Here's the drawing with two shaded views (mm, measured from the low corner). I have some questions. Give positions to 0.01 mm unless a question says otherwise; leave off trailing zeros. Order: outer loops, then holes, each group sorted by start corner. A loop starts at its lowest first (then second) coordinate and runs counter-clockwise, first axis right, second up. Notation, with made-up numbers: M -28,-38 L 19,-38 A26 cw 19,-11 Z; hole C -36.75,32 d11. An arc over 180 degrees is marked long. One line per question, with ' | ' between items. Start each with the question number.
1) If we section it at C-C, the plane y = 59.5: Please give me the cut outline in (x, z) (3 decimals), plus the area to 3 significant figures.
2) Please list where these lines run through material, in increasing order: line 1 along Y through (x, z) = (2.85, 89); line 2 along Z through (x, y) = (1.4, 42). Write a range as [from, to].
3) If we section it at A-A, the plane z = 64: Please give me the cut outline in (x, y) (3 decimals).
4) If we section it at B-B, the plane x = 0.7: Please give me the cut outline in (y, z).
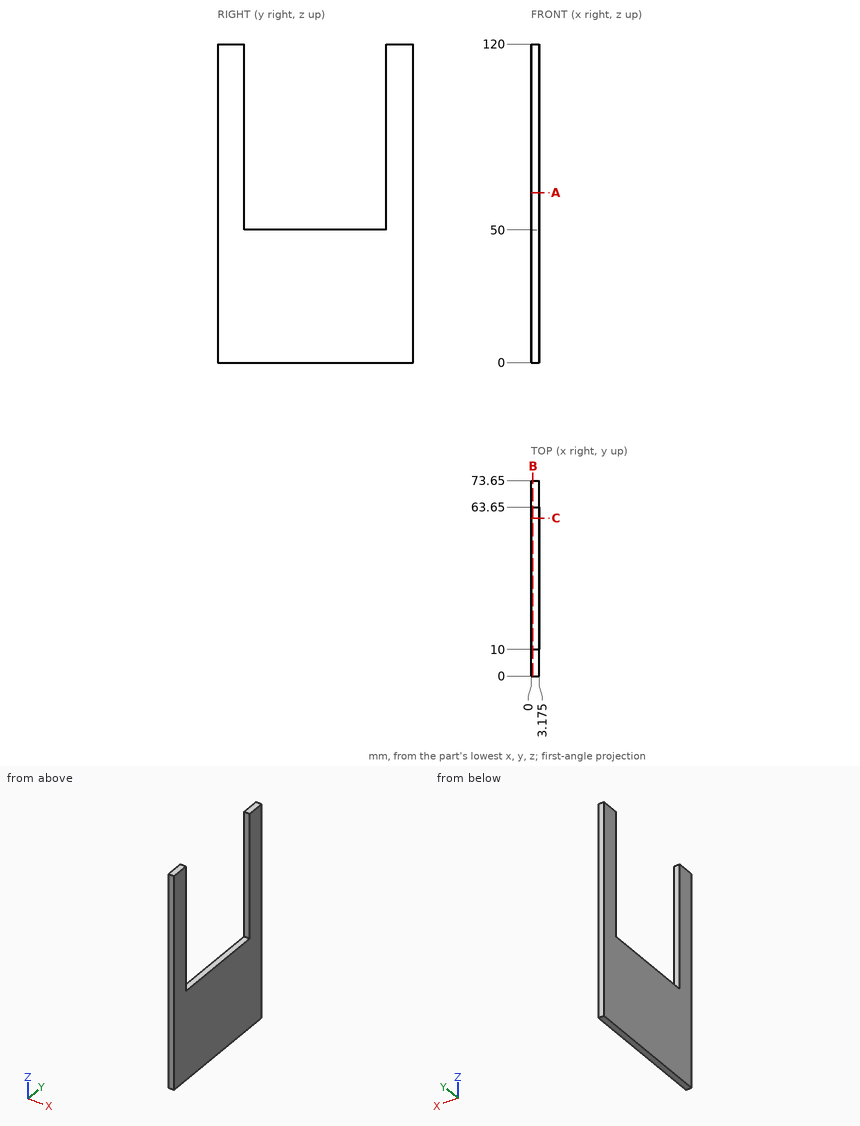
Results found:
1) outline: M 0,0 L 3.175,0 L 3.175,50 L 0,50 Z | area: 159 mm²
2) line 1: y = [0, 10], [63.65, 73.65] | line 2: z = [0, 50]
3) outline: M 0,0 L 3.175,0 L 3.175,10 L 0,10 Z; M 0,63.65 L 3.175,63.65 L 3.175,73.65 L 0,73.65 Z
4) outline: M 0,0 L 73.65,0 L 73.65,120 L 63.65,120 L 63.65,50 L 10,50 L 10,120 L 0,120 Z
